Input: part model. Units: mm. Frame: model coordinates. A direction names the side the tool comes from. Give positions to 0.01 mm unless a question says otherwise; leave off trailing zeros. Loops run counter-clockwise (first coordinate to the right, second up) from the corner with the lowest first, then second, coordinate; pieces in that order, holes last.
from build123d import *

# Parameters (mm, degrees)
SKETCH_3_R          = 12.5
SHELL_7_T           = 2
CUT_EXTRUDE_4_DEPTH = 476.300168318
SKETCH_19_R         = 7.5
CUT_EXTRUDE_5_DEPTH = 25


with BuildPart() as part:
    # 掃出5: sweep along a path in 草圖1
    with BuildLine(Plane.XY) as sweep_5_path:
        Line((0, 0), (360, 0))
        ThreePointArc((360, 0), (395.355339059, 14.644660941), (410, 50))
        Line((410, 50), (410, 240))
    # 草圖3 → 掃出5 (sweep)
    with BuildSketch(Plane(origin=(60, 240, 0), x_dir=(1, 0, 0), z_dir=(0, 1, 0))):
        with Locations((350, 0)):
            Circle(SKETCH_3_R)
    sweep(path=sweep_5_path.line)

    # 薄殼7
    shell_7_openings = [part.faces().sort_by_distance(p)[0] for p in [
        (0, 0, 0),
        (410, 240, 0),
    ]]
    offset(amount=SHELL_7_T, openings=shell_7_openings, kind=Kind.INTERSECTION)

    # 草圖18 → 除料-伸長4 (cut, through all)
    with BuildSketch(Plane(origin=(410, 0, 0), x_dir=(0, 0, -1), z_dir=(1, 0, 0))):
        with BuildLine():
            Line((-2, 760.068622847), (-2, 240))
            Line((-2, 240), (-2, 209))
            ThreePointArc((-2, 209), (0, 207), (2, 209))
            Line((2, 209), (2, 240))
            Line((2, 240), (2, 760.068622847))
            Line((2, 760.068622847), (2, 1800.205868541))
            Line((2, 1800.205868541), (-2, 1800.205868541))
            Line((-2, 1800.205868541), (-2, 760.068622847))
        make_face()
    extrude(amount=CUT_EXTRUDE_4_DEPTH, mode=Mode.SUBTRACT)

    # 草圖19 → 除料-伸長5 (cut, symmetric)
    with BuildSketch(Plane(origin=(0, 0, 0), x_dir=(1, 0, 0), z_dir=(0, 1, 0))):
        with Locations(Location((15, 0, 0), (0, 0, 270))):
            Circle(SKETCH_19_R)
    extrude(amount=CUT_EXTRUDE_5_DEPTH, both=True, mode=Mode.SUBTRACT)


solid = part.part
(1) Cut plane A-A (x = 15). Return the cut outline in (y, z), and give its area (3 significant figures).
Values follow:
outline: (-12.41, -7.5) arc R14.5 ccw to (12.41, -7.5) - (10, -7.5) arc R12.5 cw to (-10, -7.5) - close; (-12.41, 7.5) - (-10, 7.5) arc R12.5 cw to (10, 7.5) - (12.41, 7.5) arc R14.5 ccw to start
area: 106 mm2
(2) Pin query (flat end, axial travel): pin 1 Ø1.5 at (y, z) = (18, -2.5) entering from +X; pin 2 Ø5 at (y, z) = (178.5, 3.5) entering from -X; pin 3 Ø12 at (y, z) = (23.5, -7.5) entering from +X. Return the tip coordinate at first contact, or that it passes through.
Values follow:
pin 1: stops at x = 416.2
pin 2: stops at x = 395.53
pin 3: stops at x = 420.17
(3) Cut plane C-C (y = 134.5). Return the cut outline in (x, z).
Values follow:
outline: circle Ø29 at (410, 0); hole circle Ø25 at (410, 0)
(4) Reachability of faces 1 (the cylindrical face through (182.52, -11.923, -3.755)), 2 (the flat face through (414.3, 240, -11.9)), 3 (the cylindrical face through (421.923, 146.33, -3.755)) from +Z, -Z, +X, -X, +Y, -Y: full face, straight path, thin tool, end or side. Return the list, or none.
Values follow:
face 1: -X
face 2: +Z, -Z, +X, -X, +Y
face 3: +Y
(5) Ray query, probe 1 along X at (y, z) = (202.5, 1.5); probe 2 along X at (y, z) = (141, 1); probe 3 along Z at (x, y) = (84, 0). Return the intervals inside material, ascending.
Values follow:
probe 1: x = 395.58 to 397.59, 422.41 to 424.42
probe 2: x = 395.53 to 397.54, 422.46 to 424.47
probe 3: z = -14.5 to -12.5, 12.5 to 14.5
(6) Cut plane D-D (x = 164.5). Return the cut outline in (y, z).
Values follow:
outline: circle Ø29 at (0, 0); hole circle Ø25 at (0, 0)
(7) Mould query, pull axis X, two halves, no side actions, for faces 4 (the flat face through (0, -7, -11)), 5 (the cylindrical face through (423.83, 146.33, -4.36)), 6 (the cylindrical face through (20.1, 12.3, -5.5)). Classes: +X half, -X half, draft (parallel to the pull), parting line (faces both ways), or undercut.
Values follow:
face 4: -X half
face 5: parting line
face 6: undercut
(8) Cut plane B-B (y = 216). Return the cut outline in (x, z), and give its area (3 significant figures).
Values follow:
outline: (422.34, -2) arc R12.5 cw (long way) to (422.34, 2) - (424.36, 2) arc R14.5 ccw (long way) to (424.36, -2) - close
area: 162 mm2
